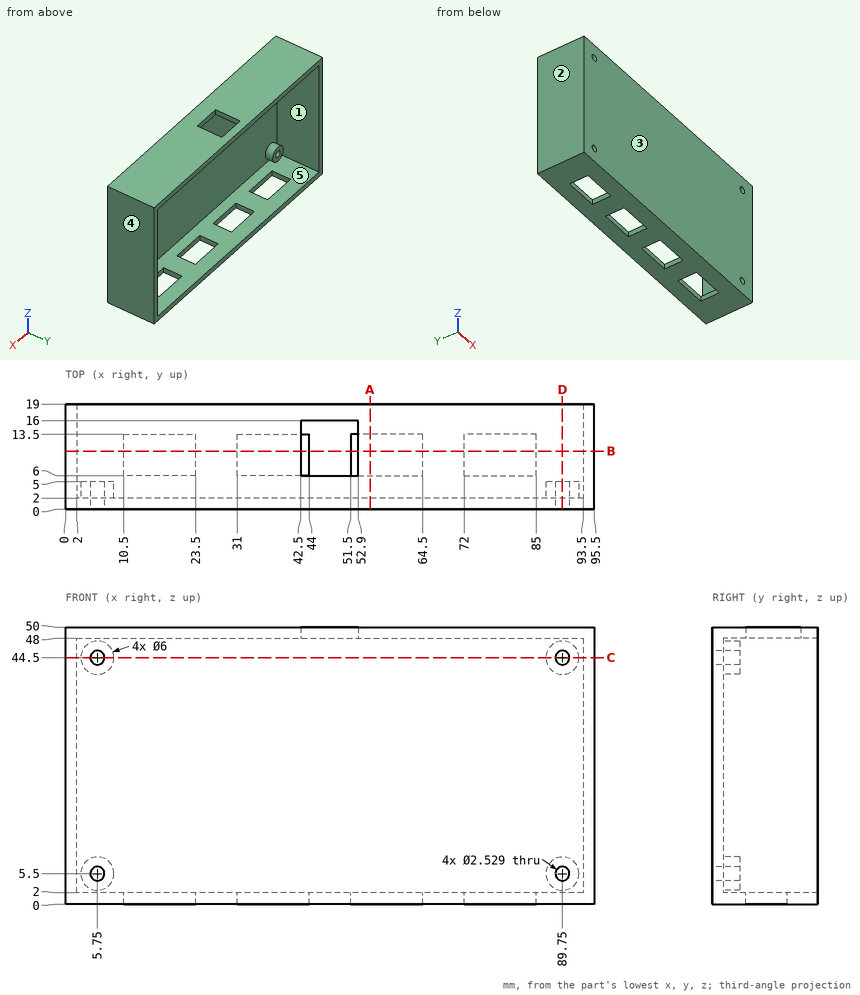
Study the drawing (mm; zero at the part's minimum x, y, z) and answer. A direction names the side the tool comes from. Give positions to 0.01 mm unless a question says otherwise; leave off trailing zeros. Order: outer loops, then holes, each group sorted by start corner. A loop starts at its lowest first (then second) coordinate and runs counter-clockwise, first axis right, second up. Notation, with made-up numbers: M 18.25,65.25 L 63.25,65.25 A14 cw 63.25,77.25 Z; hole C 10,-13.5 d9. An arc over 180 degrees is marked long. Put each result on its own line as item: value. Start each with the question number.
Item 1: For a pull along X with two mould halves and no side action, classify the marked faces 3, 4 and 5 as +X half, -X half, draft (parallel to the pull), parting line (faces both ways), or undercut.
Item 2: The part is cut by section B-B, the plane y = 10.5. Determine the outline of the cut face in (x, z).
Item 3: The part is cut by section C-C, the plane z = 44.5. Determine the outline of the cut face in (x, y).
Item 4: Which of the six approach directions +Z, -Z, +X, -X, +Y, -Y give full straight-line access (tool end or side, diameter ignored) to the marked faces 1 and 2?
Item 5: Flat-ended cylindrical pins translate along their axes: P1, Ø2, axis at x = 50.5, y = 6.5, coming from the +Z side; P2, Ø4, axis at x = 89.75, z = 5.5, coming from the +Y side; P3, Ø8, axis at x = 55.5, z = 23.5, coming from the +Y side. Find the tip coordinate at first contact, or state that the pin passes through.
Item 6: The part is cut by section D-D, the plane x = 89.75. Determine the outline of the cut face in (y, z).
Item 7: Find the intervals of material crossed by line 1 along X through (y, z) = (1.6, 5.5); line 2 along Z through (x, y) = (5.75, 2.8); line 3 along Z through (x, y) = (89.75, 1.1), in increasing order.
Item 8: The part is cut by section A-A, the plane x = 55. Determine the outline of the cut face in (y, z).
Answer key:
1. face 3: draft
1. face 4: +X half
1. face 5: undercut
2. outline: M 0,0 L 10.5,0 L 10.5,2 L 2,2 L 2,48 L 42.5,48 L 42.5,50 L 0,50 Z; M 23.5,0 L 31,0 L 31,2 L 23.5,2 Z; M 44,0 L 51.5,0 L 51.5,2 L 44,2 Z; M 52.9,48 L 93.5,48 L 93.5,2 L 85,2 L 85,0 L 95.5,0 L 95.5,50 L 52.9,50 Z; M 64.5,0 L 72,0 L 72,2 L 64.5,2 Z
3. outline: M 0,0 L 4.49,0 L 4.49,5 L 2.75,5 L 2.75,2 L 2,2 L 2,19 L 0,19 Z; M 7.01,0 L 88.49,0 L 88.49,5 L 86.75,5 L 86.75,2 L 8.75,2 L 8.75,5 L 7.01,5 Z; M 91.01,0 L 95.5,0 L 95.5,19 L 93.5,19 L 93.5,2 L 92.75,2 L 92.75,5 L 91.01,5 Z
4. face 1: +Y
4. face 2: +Z, -Z, -X, +Y, -Y
5. P1: stops at z = 50
5. P2: stops at y = 5
5. P3: stops at y = 2
6. outline: M 0,0 L 19,0 L 19,2 L 2,2 L 2,2.5 L 5,2.5 L 5,4.24 L 0,4.24 Z; M 0,6.76 L 5,6.76 L 5,8.5 L 2,8.5 L 2,41.5 L 5,41.5 L 5,43.24 L 0,43.24 Z; M 0,45.76 L 5,45.76 L 5,47.5 L 2,47.5 L 2,48 L 19,48 L 19,50 L 0,50 Z
7. line 1: x = 0 to 4.49, 7.01 to 88.49, 91.01 to 95.5
7. line 2: z = 0 to 2, 2.5 to 4.24, 6.76 to 8.5, 41.5 to 43.24, 45.76 to 47.5, 48 to 50
7. line 3: z = 0 to 4.24, 6.76 to 43.24, 45.76 to 50
8. outline: M 0,0 L 6,0 L 6,2 L 2,2 L 2,48 L 19,48 L 19,50 L 0,50 Z; M 13.5,0 L 19,0 L 19,2 L 13.5,2 Z
